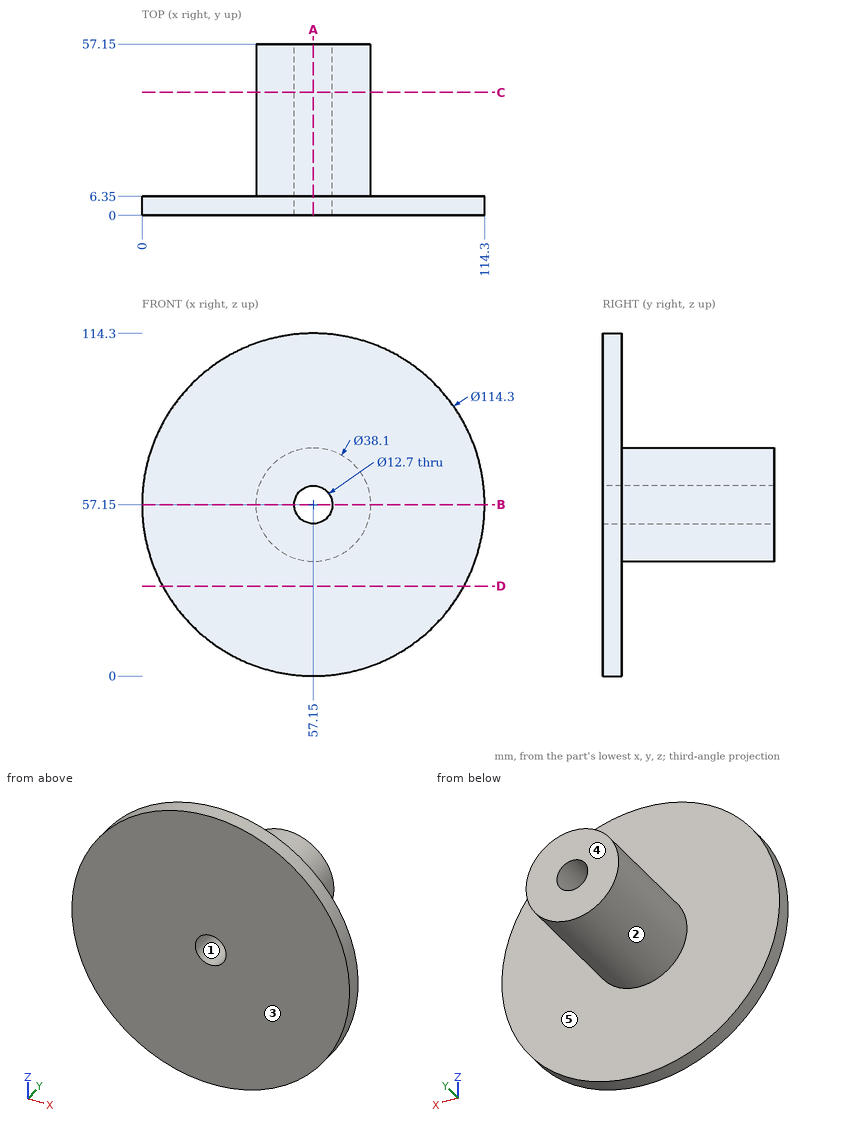
Could you check a few things on this drawing? It's one solid part, dimensions in mm from its lowest x, y, z. A direction names the side the tool comes from. Give positions to 0.01 mm unless a question says otherwise; leave off trailing zeros. Loops run counter-clockwise (first coordinate to the right, second up) from the corner with the lowest first, then second, coordinate; pieces in that order, holes last. Notation, with made-up numbers: (82, 86.5) -> (133, 86.5) arc R9 cw to (133, 90.5) -> close; hole circle Ø1 at (-30.75, -10). An arc over 180 degrees is marked (long way). Use one line per item in the form item = value. Start each with the question number.
1) Which directions (+Z, -Z, +X, -X, +Y, -Y) give clear straight access to the entire face, cutting with the end or side of a thin tool? Please do the marked faces 4 and 5.
2) Thinking about a two-plate mould opening in X: for the marked faces 1, 2 and 3, which applies, +X half, -X half, draft (parallel to the pull), parting line (faces both ways), or undercut?
3) Imagine slicing it at D-D (z = 30). Please give me the cut outline in (x, y), then the cut area to 3 significant figures.
4) For P1, Ø5, axis at y = 10, z = 58, coming from the +X side; P2, Ø10, axis at y = 27, z = 68.5, coming from the -X side; P3, Ø2, axis at x = 35.5, y = 44, coming from the -Z side; P4, Ø1, axis at x = 85, z = 71, coming from the +Y side, each with a flat end and sliding along its axis, tell me the tip position at first contact or that it passes through.
5) Imagine slicing it at C-C (y = 41). Please give me the cut outline in (x, z).
6) Imagine slicing it at B-B (z = 57.15). Please give me the cut outline in (x, y), then the cut area to 3 significant figures.
7) Imagine slicing it at A-A (x = 57.15). Please give me the cut outline in (y, z).
8) Please list where these lines run through material, in increasing order: line 1 along X through (y, z) = (37, 57.15); line 2 along Y through (x, z) = (30, 25); line 3 along Z through (x, y) = (58.5, 50).
Check values:
q1.face_4 = +Z, -Z, +X, -X, +Y
q1.face_5 = +Y
q2.face_1 = undercut
q2.face_2 = parting line
q2.face_3 = draft
q3.outline = (6.86, 0) -> (107.44, 0) -> (107.44, 6.35) -> (6.86, 6.35) -> close
q3.area = 639 mm^2
q4.P1 = 76.2
q4.P2 = 39.19
q4.P3 = through
q4.P4 = 6.35
q5.outline = circle Ø38.1 at (57.15, 57.15); hole circle Ø12.7 at (57.15, 57.15)
q6.outline = (0, 0) -> (50.8, 0) -> (50.8, 57.15) -> (38.1, 57.15) -> (38.1, 6.35) -> (0, 6.35) -> close; (63.5, 0) -> (114.3, 0) -> (114.3, 6.35) -> (76.2, 6.35) -> (76.2, 57.15) -> (63.5, 57.15) -> close
q6.area = 1,940 mm^2
q7.outline = (0, 0) -> (6.35, 0) -> (6.35, 38.1) -> (57.15, 38.1) -> (57.15, 50.8) -> (0, 50.8) -> close; (0, 63.5) -> (57.15, 63.5) -> (57.15, 76.2) -> (6.35, 76.2) -> (6.35, 114.3) -> (0, 114.3) -> close
q8.line_1 = 38.1 to 50.8, 63.5 to 76.2
q8.line_2 = 0 to 6.35
q8.line_3 = 38.15 to 50.95, 63.35 to 76.15
